```python
from build123d import *

# Parameters (mm, degrees)
SCHIZZO1_R                   = 42.562660939
ESTRUSIONE_ESTRUSIONE1_DEPTH = 5
SCHIZZO3_R                   = 11
TAGLIO_ESTRUSIONE2_DEPTH     = 6
SCHIZZO4_R                   = 1.5
SCHIZZO4_W                   = 5
SCHIZZO4_H                   = 10
SCHIZZO4_W_2                 = 10
SCHIZZO4_H_2                 = 5
TAGLIO_ESTRUSIONE3_DEPTH     = 6


with BuildPart() as part:
    # Schizzo1 → Estrusione-Estrusione1 (new body)
    with BuildSketch(Plane.XY):
        Circle(SCHIZZO1_R)
    extrude(amount=ESTRUSIONE_ESTRUSIONE1_DEPTH)

    # Schizzo3 → Taglio-Estrusione2 (cut, through all)
    with BuildSketch(Plane.XY):
        Circle(SCHIZZO3_R)
    extrude(amount=TAGLIO_ESTRUSIONE2_DEPTH, mode=Mode.SUBTRACT)

    # Schizzo4 → Taglio-Estrusione3 (cut, through all)
    with BuildSketch(Plane.XY):
        with Locations((0, 25)):
            Circle(SCHIZZO4_R)
        with Locations((17.67766953, 17.67766953)):
            Circle(SCHIZZO4_R)
        with Locations((25, 0)):
            Circle(SCHIZZO4_R)
        with Locations((17.67766953, -17.67766953)):
            Circle(SCHIZZO4_R)
        with Locations((0, -25)):
            Circle(SCHIZZO4_R)
        with Locations((-17.67766953, -17.67766953)):
            Circle(SCHIZZO4_R)
        with Locations((-25, 0)):
            Circle(SCHIZZO4_R)
        with Locations((-17.67766953, 17.67766953)):
            Circle(SCHIZZO4_R)
        with Locations((-25, -10)):
            Rectangle(SCHIZZO4_W, SCHIZZO4_H)
        with Locations((-25, 10)):
            Rectangle(SCHIZZO4_W, SCHIZZO4_H)
        with Locations((10, 25)):
            Rectangle(SCHIZZO4_W_2, SCHIZZO4_H_2)
        with Locations((-10, 25)):
            Rectangle(SCHIZZO4_W_2, SCHIZZO4_H_2)
        with Locations((25, -10)):
            Rectangle(SCHIZZO4_W, SCHIZZO4_H)
        with Locations((25, 10)):
            Rectangle(SCHIZZO4_W, SCHIZZO4_H)
        with Locations((-10, -25)):
            Rectangle(SCHIZZO4_W_2, SCHIZZO4_H_2)
        with Locations((10, -25)):
            Rectangle(SCHIZZO4_W_2, SCHIZZO4_H_2)
    extrude(amount=TAGLIO_ESTRUSIONE3_DEPTH, mode=Mode.SUBTRACT)


solid = part.part
```
CAD build for the part. Positions are in the model's coordinates, mm. Round coordinates to 2 decimals unless told otherwise and drop trailing zeros. Order: outer loops, then holes, each group sorted by start corner. A loop starts at its lowest first (then second) coordinate and runs counter-clockwise, first axis right, second up. Notation, with made-up numbers: (-12.75, -39) -> (-6.75, -39) arc R21 cw to (-6.75, -2) -> close; hole circle Ø6 at (-16.5, -22). An arc over 180 degrees is marked (long way). Write item = value, one per line.
(1) Pull direction Y, two halves, no side cores. Call faces 1 (the cylindrical face through (-9.23, -41.55, 2.46)), 2 (the flat face through (-15, 25, 2)), 3 (the flat face through (-10, -27.5, 2)): +Y half, -Y half, draft (parallel to the pull), parting line (faces both ways), or undercut.
Answers follow:
face_1 = parting line
face_2 = undercut
face_3 = undercut
(2) Drill centre lines: L1, parallel to Y at x = 0, z = 1.6; L2, parallel to Y at x = -25, z = 2.8; L3, parallel to Y at x = -27, z = 4.35. Where is each one in solid material? Low to high.
Answers follow:
L1 = -42.56 to -26.5, -23.5 to -11, 11 to 23.5, 26.5 to 42.56
L2 = -34.45 to -15, -5 to -1.5, 1.5 to 5, 15 to 34.45
L3 = -32.9 to -15, -5 to 5, 15 to 32.9
(3) Flat gauge pins, fed straight in: P1, Ø2.5, axis at y = -8, z = 1.5, coming from the +X side; P2, Ø3, axis at x = -33, z = 1.5, coming from the -Y side; P3, Ø1.5, axis at y = 24, z = 1.5, coming from the +X side. Where does each tip first touch, or does it go through?
Answers follow:
P1 = 42.02
P2 = -28.62
P3 = 35.65
(4) Cut at A-A (x = 0). Write the cut outline in (y, z).
Answers follow:
outline = (-42.56, 0) -> (-26.5, 0) -> (-26.5, 5) -> (-42.56, 5) -> close; (-23.5, 0) -> (-11, 0) -> (-11, 5) -> (-23.5, 5) -> close; (11, 0) -> (23.5, 0) -> (23.5, 5) -> (11, 5) -> close; (26.5, 0) -> (42.56, 0) -> (42.56, 5) -> (26.5, 5) -> close
(5) Cut at C-C (y = -12.5). Write the cut outline in (x, z), plus the area to 3 significant figures.
Answers follow:
outline = (-40.69, 0) -> (-27.5, 0) -> (-27.5, 5) -> (-40.69, 5) -> close; (-22.5, 0) -> (22.5, 0) -> (22.5, 5) -> (-22.5, 5) -> close; (27.5, 0) -> (40.69, 0) -> (40.69, 5) -> (27.5, 5) -> close
area = 357 mm²
(6) Cut at D-D (x = 13.5). Write the cut outline in (y, z), plus the area to 3 significant figures.
Answers follow:
outline = (-40.36, 0) -> (-27.5, 0) -> (-27.5, 5) -> (-40.36, 5) -> close; (-22.5, 0) -> (22.5, 0) -> (22.5, 5) -> (-22.5, 5) -> close; (27.5, 0) -> (40.36, 0) -> (40.36, 5) -> (27.5, 5) -> close
area = 354 mm²
